```python
from build123d import *

# Parameters (mm, degrees)
SKETCH1_W                     = 241.3
SKETCH1_H                     = 241.3
BOSS_EXTRUDE1_DEPTH           = 25.4
BOSS_EXTRUDE2_DEPTH           = 38.1
BOSS_EXTRUDE3_START           = -38.1
BOSS_EXTRUDE3_DEPTH           = 38.1
F_1_1_8_CLEARANCE_HOLE1_D     = 29.45892
F_1_1_8_CLEARANCE_HOLE1_DEPTH = 177.8
F_1_1_8_CLEARANCE_HOLE2_D     = 29.45892
SKETCH8_W                     = 38.1
SKETCH8_H                     = 82.55
HOLE2_D                       = 76.2
HOLE2_DEPTH                   = 82.55
CHAMFER1_SIZE                 = 1.14554


with BuildPart() as part:
    # Sketch1 → Boss-Extrude1 (new body)
    with BuildSketch(Plane(origin=(25.4, 0, 0), x_dir=(0, 0, -1), z_dir=(1, 0, 0))):
        Rectangle(SKETCH1_W, SKETCH1_H)
    extrude(amount=-BOSS_EXTRUDE1_DEPTH)

    # Sketch2 → Boss-Extrude2 (add)
    with BuildSketch(Plane(origin=(0, 0, -76.2), x_dir=(-1, 0, 0), z_dir=(0, 0, -1))):
        with BuildLine():
            Line((-25.4, -69.85), (-25.4, 69.85))
            Line((-25.4, 69.85), (-107.95, 69.85))
            ThreePointArc((-107.95, 69.85), (-177.8, 0), (-107.95, -69.85))
            Line((-107.95, -69.85), (-25.4, -69.85))
        make_face()
    extrude(amount=-BOSS_EXTRUDE2_DEPTH)

    # Sketch3 → Boss-Extrude3 (add)
    with BuildSketch(Plane.XY.offset(76.2).offset(BOSS_EXTRUDE3_START)):
        with BuildLine():
            Line((25.4, 69.85), (25.4, -69.85))
            Line((25.4, -69.85), (107.95, -69.85))
            ThreePointArc((107.95, -69.85), (177.8, 0), (107.95, 69.85))
            Line((107.95, 69.85), (25.4, 69.85))
        make_face()
    extrude(amount=BOSS_EXTRUDE3_DEPTH)

    # 1-1/8 Clearance Hole1
    with Locations(Plane.ZY):
        with Locations((-95.25, -95.25), (95.25, -95.25)):
            Hole(F_1_1_8_CLEARANCE_HOLE1_D / 2, depth=F_1_1_8_CLEARANCE_HOLE1_DEPTH)

    # 1-1/8 Clearance Hole2 (through all)
    with Locations(Plane(origin=(25.4, 0, 0), x_dir=(0, 0, -1), z_dir=(1, 0, 0))):
        with Locations((-95.25, 95.25), (95.25, 95.25)):
            Hole(F_1_1_8_CLEARANCE_HOLE2_D / 2)

    # Sketch8 → Hole1 (revolve, cut)
    with BuildSketch(Plane(origin=(107.95, 0, 38.1), x_dir=(0, 1, 0), z_dir=(1, 0, 0))):
        with Locations((19.05, 41.275)):
            Rectangle(SKETCH8_W, SKETCH8_H)
    revolve(axis=Axis((107.95, 0, 148.1), (0, 0, -1)), mode=Mode.SUBTRACT)

    # Hole2
    with Locations(Plane.XY.offset(-38.1)):
        with Locations((107.95, 0)):
            Hole(HOLE2_D / 2, depth=HOLE2_DEPTH)

    # Chamfer1
    chamfer1_edges = [part.edges().sort_by_distance(p)[0] for p in [
        (25.4, -95.25, 109.97946),
        (0, -95.25, 109.97946),
        (25.4, -95.25, -80.52054),
        (0, -95.25, -80.52054),
        (25.4, 95.25, -109.97946),
        (0, 95.25, -109.97946),
        (25.4, 95.25, 80.52054),
        (0, 95.25, 80.52054),
    ]]
    chamfer(chamfer1_edges, length=CHAMFER1_SIZE)


solid = part.part
```
Build history of the part. All positions in model axes, mm. A direction names the side the tool comes from. Give positions to 0.01 mm unless a question says otherwise; leave off trailing zeros. Loops run counter-clockwise (first coordinate to the right, second up) from the corner with the lowest first, then second, coordinate; pieces in that order, holes last.
1) Drop flat-ended pins along their axis: P1, Ø17.5, axis at y = -95.25, z = -95.25, coming from the -X side; P2, Ø11.5, axis at x = 50, z = -55.5, coming from the +Y side; P3, Ø8, axis at x = 44, y = 25, coming from the -Z side; P4, Ø1.5, axis at x = 104.5, y = -45, coming from the +Z side. Give the stop position or say it passes through.
Values follow:
P1: passes through
P2: stops at y = 69.85
P3: stops at z = -76.2
P4: stops at z = 76.2
2) Two-plate mould, pull along Y, no slides. Class faces 4 (the face through (13, 120.65, 2)), 5 (the face through (67, -69.85, -57)), 6 (the face through (12.538, 109.854, -97.167)): released by +Y, released by -Y, zero draft, split by the parting line, or undercut.
Values follow:
face 4: released by +Y
face 5: released by -Y
face 6: undercut
3) Probe line 1 along Y through (x, z) = (17.5, -95.25); line 2 along Y through (x, z) = (107.95, -63.5). List the from-to ranges inside material, lowest first.
Values follow:
line 1: y = -120.65 to -109.98, -80.52 to 80.52, 109.98 to 120.65
line 2: y = -69.85 to -38.1, 38.1 to 69.85
4) Band-saw the part on C-C on z = 62.5. List the corners of the cut face in (x, y).
Values follow:
outline: (0, -120.65) - (25.4, -120.65) - (25.4, -69.85) - (107.95, -69.85) arc R69.85 ccw to (107.95, 69.85) - (25.4, 69.85) - (25.4, 120.65) - (0, 120.65) - close; hole circle Ø76.2 at (107.95, 0)
5) Band-saw the part on D-D on x = 116. List the corners of the cut face in (y, z), then the cut area to 3 significant figures.
Values follow:
outline: (-69.38, -76.2) - (-37.24, -76.2) - (-37.24, -38.1) - (-69.38, -38.1) - close; (-69.38, 38.1) - (-37.24, 38.1) - (-37.24, 76.2) - (-69.38, 76.2) - close; (37.24, -76.2) - (69.38, -76.2) - (69.38, -38.1) - (37.24, -38.1) - close; (37.24, 38.1) - (69.38, 38.1) - (69.38, 76.2) - (37.24, 76.2) - close
area: 4,900 mm2
6) 3-axis set-ups, long thin cutter, end or side, ignore diameter. For faces 1 (the face through (67, 1, 38.1)), 2 (the face through (69, 1, -76.2)), 3 (the face through (66, -69.85, 57)): which of +Z, -Z, +X, -X, +Y, -Y reach the whole face in a straight line?
Values follow:
face 1: +X, +Y, -Y
face 2: -Z, +X, +Y, -Y
face 3: +Z, -Z, +X, -Y
7) Band-saw the part on B-B on y = 0. List the corners of the cut face in (x, z), then the cut area to 3 significant figures.
Values follow:
outline: (0, -120.65) - (25.4, -120.65) - (25.4, -76.2) - (69.85, -76.2) - (69.85, -38.1) - (25.4, -38.1) - (25.4, 38.1) - (69.85, 38.1) - (69.85, 76.2) - (25.4, 76.2) - (25.4, 120.65) - (0, 120.65) - close; (146.05, -76.2) - (177.8, -76.2) - (177.8, -38.1) - (146.05, -38.1) - close; (146.05, 38.1) - (177.8, 38.1) - (177.8, 76.2) - (146.05, 76.2) - close
area: 11,900 mm2
8) Band-saw the part on A-A on z = 95.25. List the corners of the cut face in (x, y) (3 decimals), then the cut area to 3 significant figures.
Values follow:
outline: (0, -120.65) - (25.4, -120.65) - (25.4, -111.125) - (24.254, -109.979) - (1.146, -109.979) - (0, -111.125) - close; (0, -79.375) - (1.146, -80.521) - (24.254, -80.521) - (25.4, -79.375) - (25.4, 79.375) - (24.254, 80.521) - (1.146, 80.521) - (0, 79.375) - close; (0, 111.125) - (1.146, 109.979) - (24.254, 109.979) - (25.4, 111.125) - (25.4, 120.65) - (0, 120.65) - close
area: 4,630 mm2
